Geometry check sheet. Reference: the model listing, model coordinates, mm. A direction names the side the tool comes from. Give positions to 0.01 mm unless a question says otherwise; leave off trailing zeros. Order: outer loops, then holes, each group sorted by start corner. A loop starts at its lowest first (then second) coordinate and runs counter-clockwise, first axis right, second up. Notation, with made-up numbers: M 0,-34 L 49,-34 A27 ccw 49,-4 Z; hole C -11.5,35.25 d3. An arc over 180 degrees is marked long. Answer as a JSON object with one key per item and string values. Group by question number.
Autodesk Inventor part; units mm, degrees
ref_plane "YZ Plane" through (0, 0, 0) normal (1, 0, 0) x (0, 1, 0)
ref_plane "XZ Plane" through (0, 0, 0) normal (0, 1, 0) x (-1, 0, 0)
ref_plane "XY Plane" through (0, 0, 0) normal (0, 0, 1) x (1, 0, 0)
sketch "Sketch1" plane through (0, 0, 0) normal (0, 0, 1) x (1, 0, 0)
  line L0 (0, 33.6) -> (0, -33.6)
  line L1 (-14, 0) -> (14, 0)
  line L2 (-10, 24) -> (10, 24)
  line L3 (10, 24) -> (10, -24)
  line L4 (10, -24) -> (-10, -24)
  line L5 (-10, -24) -> (-10, 24)
  point P0 (0, 0)
  dimension "d0" = 20
  dimension "d1" = 48
extrude "Extrusion1" add sketch "Sketch1" along normal blind 25
sketch "Sketch2" plane through (0, 0, 25) normal (0, 0, 1) x (1, 0, 0)
  line L0 (-10, -24) -> (10, -24)
  line L1 (10, -24) -> (10, 24)
  line L2 (10, 24) -> (-10, 24)
  line L3 (-10, 24) -> (-10, -24)
  line L4 (0, 47.04) -> (0, -47.04)
  line L5 (3, 33.6) -> (3, -33.6)
  line L6 (-3, 33.6) -> (-3, -33.6)
  point P0 (0, 0)
  point P1 (3, 24)
  point P2 (3, -24)
  point P3 (-3, -24)
  point P4 (-3, 24)
  dimension "d4" = 3
  dimension "d5" = 3
extrude "Extrusion2" cut sketch "Sketch2" against normal blind 1.5 contours L3 L2 L6 L0 | L5 L2 L1 L0
sketch "Sketch3" plane through (10, -24, 0) normal (1, 0, 0) x (0, 0, -1)
  line L0 (-30, 24) -> (5, 24)
  line L1 (-23.5, 48) -> (-23.5, 0)
  line L2 (0, 0) -> (-23.5, 0)
  line L3 (0, 0) -> (0, 48)
  line L4 (0, 48) -> (-23.5, 48)
  line L5 (-25, 0) -> (-25, 48)
  line L6 (-23.5, 0) -> (-25, 0)
  line L7 (-23.5, 0) -> (-23.5, 48)
  line L8 (-25, 48) -> (-23.5, 48)
  line L9 (0, 0) -> (-23.5, 0)
  line L10 (-11.75, 0) -> (-11.75, 48)
  line L11 (0, 48) -> (-23.5, 48)
  point P0 (0, 24)
sketch "Sketch4" plane through (10, -24, 0) normal (1, 0, 0) x (0, 0, -1)
  point P0 (0, 24)
  point P1 (-11.8566, 24.141)
hole "Hole1" at (10, 0.141, 11.8566) direction (-1, 0, 0) diameter 6.647 end through all
sketch "Sketch5" plane through (0, 0, 25) normal (0, 0, 1) x (1, 0, 0)
  line L0 (3, -24) -> (3, 24)
  line L1 (3, 24) -> (-3, 24)
  line L2 (-3, 24) -> (-3, -24)
  line L3 (-3, -24) -> (3, -24)
  circle A0 centre (0, 16) radius 3
  circle A1 centre (0, -16) radius 3
  line L4 (0, 33.6) -> (0, -33.6)
  point P0 (0, 0)
  dimension "d15" = 6
  dimension "d16" = 6
  dimension "d17" = 8
  dimension "d18" = 8
extrude "Extrusion3" cut sketch "Sketch5" against normal through all contours A1 L4 | A0 L4 | L4 A1 | L4 A0
properties part number "elbow clamp"
1. Cross-section at D-D (z = 2). Record the cut outline in (x, y), and give its area (3 significant figures).
2. Cross-section at B-B (x = 0). Record the cut outline in (y, z), and give its area (3 significant figures).
3. Cross-section at A-A (z = 10.5). Record the cut outline in (x, y), and give its area (3 significant figures).
4. Access from +Z, -Z, +X, -X, +Y, -Y to the whole of each face (thin tool, end or side, straight path). Record for faces 1 (the flat face through (6, 0, 23.5)), 2 (the flat face through (-3, 0, 24)), 3 (the flat face through (0, 0, 0)).
5. Depth check by flat-ended pin: pin 1 (1.6 mm diameter, centred on y = -18.5, z = 24, fed in from +X); pin 2 (1 mm diameter, centred on x = 6.5, y = 17.5, fed in from +Z); pin 3 (6 mm diameter, centred on y = 0.14, z = 11.86, fed in from -X); pin 4 (0.8 mm diameter, centred on y = 18.5, z = 24.5, fed in from +X). Enter the tip coordinate at first touch or a pass-through.
6. Release check for a two-part mould opening along X. For faces 4 (the cylindrical face through (-0.65, 13.07, 12.68)), 5 (the flat face through (0, -24, 12)), 6 (the flat face through (3, -20, 24)), 7 (the cylindrical face through (-0.65, -18.93, 12.68)) record: released by +X, released by -X, zero draft, split by the parting line, or undercut.
7. Cross-section at C-C (y = 10). Record the cut outline in (x, z), and give its area (3 significant figures).
8. Thickness scan on line 1 along Y through (x, z) = (0, 3.5); line 2 along X through (y, z) = (-16, 9.5); line 3 along Y through (x, z) = (0, 11.5). Record the ranges inside material, lowest first. Write a range as [from, to].
Report:
{
 "1": {"outline": "M -10,-24 L 10,-24 L 10,24 L -10,24 Z; hole C 0,-16 d6; hole C 0,16 d6", "area": "903 mm2"},
 "2": {"outline": "M -24,0 L -19,0 L -19,25 L -24,25 Z; M -13,0 L 13,0 L 13,25 L -13,25 Z; M 19,0 L 24,0 L 24,25 L 19,25 Z; hole C 0.14,11.86 d6.65", "area": "865 mm2"},
 "3": {"outline": "M -10,-24 L 10,-24 L 10,-2.89 L -10,-2.89 Z; M -10,3.18 L 10,3.18 L 10,24 L -10,24 Z; hole C 0,-16 d6; hole C 0,16 d6", "area": "782 mm2"},
 "4": {"face 1": "+Z, +X, +Y, -Y", "face 2": "+Z, -X, +Y, -Y", "face 3": "-Z, +X, -X, +Y, -Y"},
 "5": {"pin 1": "stops at x = 10", "pin 2": "stops at z = 23.5", "pin 3": "passes through", "pin 4": "stops at x = 3"},
 "6": {"face 4": "undercut", "face 5": "zero draft", "face 6": "released by +X", "face 7": "undercut"},
 "7": {"outline": "M -10,0 L 10,0 L 10,23.5 L 3,23.5 L 3,25 L -3,25 L -3,23.5 L -10,23.5 Z", "area": "479 mm2"},
 "8": {"line 1": "y = [-24, -19], [-13, 13], [19, 24]", "line 2": "x = [-10, -3], [3, 10]", "line 3": "y = [-24, -19], [-13, -3.16], [3.45, 13], [19, 24]"}
}
